Work out the finished part from the listing and answer in its coordinate system (mm). Face numbers are marked on the shaded views. Give positions to 0.01 mm unless a question says otherwise; leave off trailing zeros. Order: outer loops, then holes, each group sorted by start corner. A loop starts at its lowest first (then second) coordinate and runs counter-clockwise, first axis right, second up. Notation, with made-up numbers: (-31.5, 2) -> (27.5, 2) arc R12 ccw to (27.5, 6) -> close; hole circle Ø8 at (5.25, 40.25). An arc over 180 degrees is marked (long way). Answer as CSV lines item,"result". Start each with the question number.
1. A cutting plane is placed at D-D (x = -9). Give the vertices of the cut face in (y, z), then the cut area to 3 significant figures.
2. Flat-ended cylindrical pins translate along their axes: pin 1 (23 mm diameter, centred on x = 76, z = 94, fed in from -Y); pin 2 (3 mm diameter, centred on x = 0, y = 12, fed in from +Z); pin 3 (4 mm diameter, centred on x = 120, y = 12, fed in from +Z). Find the tip coordinate at first contact, or state that the pin passes through.
3. For a pull along X with two mould halves and no side action, classify the marked faces 1 and 2 as released by +X, released by -X, zero draft, split by the parting line, or undercut.
4. Find the intervals of material crossed by L1, parallel to Z at x = -76, y = 9; L2, parallel to X at y = 12, z = -117.25; L3, parallel to Y at x = -120, z = 120, in increasing order.
5. A cutting plane is placed at B-B (z = 60). Give the vertices of the cut face in (x, y), then the cut area to 3 significant figures.
6. A cutting plane is placed at C-C (z = 94). Give the vertices of the cut face in (x, y), then the cut area to 3 significant figures.
7. A cutting plane is placed at A-A (x = -76). Give the vertices of the cut face in (y, z), then the cut area to 3 significant figures.
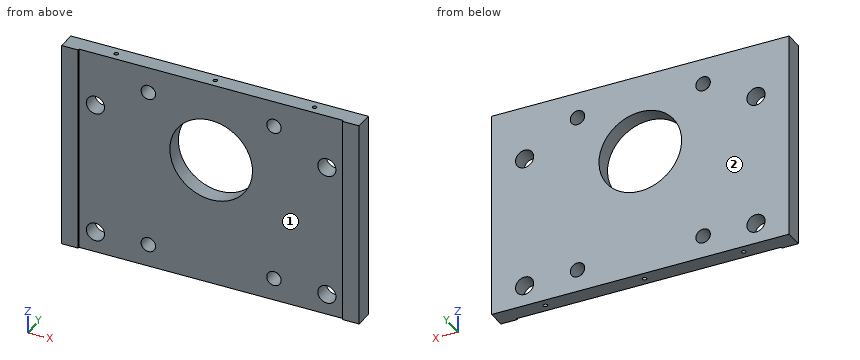
from build123d import *

# Parameters (mm, degrees)
SKETCH_1_W                  = 360
SKETCH_1_H                  = 250
EXTRUDE_1_DEPTH             = 22
CUT_EXTRUDE_1_REACH         = 222.248
SKETCH_2_R                  = 50
SKETCH_2_R_2                = 11
SKETCH_3_W                  = 320
SKETCH_3_H                  = 250
CUT_EXTRUDE_2_DEPTH         = 2
PATTERN_START               = 2
PATTERN_LINEAR_1_OUTLINE_R  = 11
PATTERN_LINEAR_1_DEPTH      = 20
HOLE_WIZARD_M20_1_D         = 17.5
PATTERN_LINEAR_2_COUNT      = 2
PATTERN_LINEAR_2_PITCH      = 192
PATTERN_LINEAR_2_COUNT_DIR2 = 2
PATTERN_LINEAR_2_PITCH_DIR2 = 152
HOLE_WIZARD_M6_1_AT_2_COUNT = 2
HOLE_WIZARD_M6_1_AT_2_PITCH = 120
HOLE_WIZARD_M6_1_AT_3_COUNT = 2
HOLE_WIZARD_M6_1_AT_3_PITCH = 240


# Read off the part's stored shape, not the designer's step: 阵列(线性)1
with BuildPart() as part:
    # 草图1 → 凸台-拉伸1 (new body)
    with BuildSketch(Plane(origin=(0, 0, 0), x_dir=(1, 0, 0), z_dir=(0, 1, 0))):
        Rectangle(SKETCH_1_W, SKETCH_1_H)
    extrude(amount=EXTRUDE_1_DEPTH)

    # 草图2 → 切除-拉伸1 (cut, up to next)
    with BuildSketch(Plane.XZ, mode=Mode.PRIVATE) as cut_extrude_1_sk1:
        with Locations(Location((0, 30, 0), (0, 0, 270))):
            Circle(SKETCH_2_R)
    cut_extrude_1_tool1 = extrude(cut_extrude_1_sk1.sketch, amount=-CUT_EXTRUDE_1_REACH, mode=Mode.PRIVATE) & part.part
    # 草图2 → 切除-拉伸1 (cut, up to next)
    with BuildSketch(Plane.XZ, mode=Mode.PRIVATE) as cut_extrude_1_sk2:
        with Locations(Location((-140, 60, 0), (0, 0, 270))):
            Circle(SKETCH_2_R_2)
    cut_extrude_1_tool2 = extrude(cut_extrude_1_sk2.sketch, amount=-CUT_EXTRUDE_1_REACH, mode=Mode.PRIVATE) & part.part
    add(cut_extrude_1_tool1.solids().sort_by_distance((0, 0, 30))[0], mode=Mode.SUBTRACT)
    add(cut_extrude_1_tool2.solids().sort_by_distance((-140, 0, 60))[0], mode=Mode.SUBTRACT)

    # 草图3 → 切除-拉伸2 (cut)
    with BuildSketch(Plane.XZ):
        Rectangle(SKETCH_3_W, SKETCH_3_H)
    extrude(amount=-CUT_EXTRUDE_2_DEPTH, mode=Mode.SUBTRACT)

    # 阵列(线性)1 outline → 阵列(线性)1 (cut)
    with BuildSketch(Plane(origin=(0, 0, 0), x_dir=(1, 0, 0), z_dir=(0, 1, 0)).offset(PATTERN_START)):
        with Locations((140, 100)):
            Circle(PATTERN_LINEAR_1_OUTLINE_R)
        with Locations((-140, 100)):
            Circle(PATTERN_LINEAR_1_OUTLINE_R)
        with Locations((140, -60)):
            Circle(PATTERN_LINEAR_1_OUTLINE_R)
    extrude(amount=PATTERN_LINEAR_1_DEPTH, mode=Mode.SUBTRACT)

    # M20 螺纹孔1 (through all)
    with Locations(Plane(origin=(0, 2, 0), x_dir=(-1, 0, 0), z_dir=(0, -1, 0))):
        with Locations((76, -94)):
            hole_wizard_m20_1 = Hole(HOLE_WIZARD_M20_1_D / 2)

    # 阵列(线性)2: Hole Wizard M20 _1 2 × 2
    with Locations(*[(j * PATTERN_LINEAR_2_PITCH_DIR2, 0, -i * PATTERN_LINEAR_2_PITCH) for i in range(PATTERN_LINEAR_2_COUNT) for j in range(PATTERN_LINEAR_2_COUNT_DIR2) if (i, j) != (0, 0)]):
        add(hole_wizard_m20_1, mode=Mode.SUBTRACT)

    # 草图7 → M6 螺纹孔1 (revolve, cut)
    with BuildSketch(Plane(origin=(120, 12, -125), x_dir=(0, 1, 0), z_dir=(1, 0, 0))):
        Polygon((0, 0), (0, 16.502151548), (2.5, 15), (2.5, 0), align=None)
    hole_wizard_m6_1 = revolve(axis=Axis((120, 12, -131.35), (0, 0, 1)), mode=Mode.SUBTRACT)

    # M6 螺纹孔1 at 2: M6 螺纹孔1 ×2
    with Locations(*[(-i * HOLE_WIZARD_M6_1_AT_2_PITCH, 0, 0) for i in range(1, HOLE_WIZARD_M6_1_AT_2_COUNT)]):
        add(hole_wizard_m6_1, mode=Mode.SUBTRACT)

    # M6 螺纹孔1 at 3: M6 螺纹孔1 ×2
    with Locations(*[(-i * HOLE_WIZARD_M6_1_AT_3_PITCH, 0, 0) for i in range(1, HOLE_WIZARD_M6_1_AT_3_COUNT)]):
        add(hole_wizard_m6_1, mode=Mode.SUBTRACT)

    # 镜向1: M6 螺纹孔1 across plane
    add(hole_wizard_m6_1.mirror(Plane.XY), mode=Mode.SUBTRACT)

    # 镜向1 copy 1 sketch → 镜向1 copy 1 (revolve, cut)
    with BuildSketch(Plane(origin=(0, 12, 125), x_dir=(0, 1, 0), z_dir=(1, 0, 0))):
        Polygon((0, 0), (0, -16.502151548), (2.5, -15), (2.5, 0), align=None)
    revolve(axis=Axis((0, 12, 131.35), (0, 0, 1)), mode=Mode.SUBTRACT)

    # 镜向1 copy 2 sketch → 镜向1 copy 2 (revolve, cut)
    with BuildSketch(Plane(origin=(-120, 12, 125), x_dir=(0, 1, 0), z_dir=(1, 0, 0))):
        Polygon((0, 0), (0, -16.502151548), (2.5, -15), (2.5, 0), align=None)
    revolve(axis=Axis((-120, 12, 131.35), (0, 0, 1)), mode=Mode.SUBTRACT)


solid = part.part
Answer sheet:
1,outline,"(2, -125) -> (22, -125) -> (22, -19.18) -> (2, -19.18) -> close; (2, 79.18) -> (22, 79.18) -> (22, 125) -> (2, 125) -> close"
1,area,"3,030 mm^2"
2,pin 1,"stops at y = 2"
2,pin 2,"stops at z = 109.4"
2,pin 3,"stops at z = 109.7"
3,face 1,"undercut"
3,face 2,"zero draft"
4,L1,"z = -125 to -106.75, -89.25 to 85.25, 102.75 to 125"
4,L2,"x = -180 to -122.5, -117.5 to -2.5, 2.5 to 117.5, 122.5 to 180"
4,L3,"y = 2 to 9.5, 14.5 to 22"
5,outline,"(-180, 0) -> (-160, 0) -> (-160, 2) -> (-151, 2) -> (-151, 22) -> (-180, 22) -> close; (-129, 2) -> (-40, 2) -> (-40, 22) -> (-129, 22) -> close; (40, 2) -> (129, 2) -> (129, 22) -> (40, 22) -> close; (151, 2) -> (160, 2) -> (160, 0) -> (180, 0) -> (180, 22) -> (151, 22) -> close"
5,area,"4,800 mm^2"
6,outline,"(-180, 0) -> (-160, 0) -> (-160, 2) -> (-84.75, 2) -> (-84.75, 22) -> (-180, 22) -> close; (-67.25, 2) -> (67.25, 2) -> (67.25, 22) -> (-67.25, 22) -> close; (84.75, 2) -> (160, 2) -> (160, 0) -> (180, 0) -> (180, 22) -> (84.75, 22) -> close"
6,area,"6,580 mm^2"
7,outline,"(2, -125) -> (22, -125) -> (22, -106.75) -> (2, -106.75) -> close; (2, -89.25) -> (22, -89.25) -> (22, 85.25) -> (2, 85.25) -> close; (2, 102.75) -> (22, 102.75) -> (22, 125) -> (2, 125) -> close"
7,area,"4,300 mm^2"
